Autodesk Inventor part; units mm, degrees
ref_plane "YZ Plane" through (0, 0, 0) normal (1, 0, 0) x (0, 1, 0)
ref_plane "XZ Plane" through (0, 0, 0) normal (0, 1, 0) x (-1, 0, 0)
ref_plane "XY Plane" through (0, 0, 0) normal (0, 0, 1) x (1, 0, 0)
sketch "Skizze1" plane through (0, 0, 0) normal (0, 0, 1) x (1, 0, 0)
  line L0 (-1.4434, 2.5) -> (1.4434, 2.5)
  line L1 (1.4434, 2.5) -> (2.8868, 0)
  line L2 (2.8868, 0) -> (1.4434, -2.5)
  line L3 (1.4434, -2.5) -> (-1.4434, -2.5)
  line L4 (-1.4434, -2.5) -> (-2.8868, 0)
  line L5 (-2.8868, 0) -> (-1.4434, 2.5)
  point P0 (0, 0)
  point P1 (0, 0)
  point P2 (0, 2.5)
  point P3 (0, -2.5)
  dimension "d3" = 120
  dimension "d4" = 120
  dimension "d5" = 120
  dimension "d6" = 5
extrude "Extrusion1" add sketch "Skizze1" along normal blind 5
sketch "Skizze2" plane through (0, 0, 5) normal (0, 0, 1) x (1, 0, 0)
  point P0 (0, 0)
  point P1 (0, 0)
hole "Bohrung1" at (0, 0, 5) direction (0, 0, -1) diameter 2.5 depth 4 tip angle 118
thread "Gewinde1"
sketch "Skizze3" plane through (0, 0, 0) normal (0, 0, -1) x (-1, 0, 0)
  circle A0 centre (0, 0) radius 1.25
  dimension "d18" = 2.5
extrude "Extrusion2" add sketch "Skizze3" along normal blind 4
thread "Gewinde2"
properties part number "5mm_Außengewinde"
CAD build for the part. Positions are in the model's coordinates, mm. A direction names the side the tool comes from. Coordinates: 2 decimals unless noted, no trailing zeros. Loops run counter-clockwise (first coordinate to the right, second up) from the corner with the lowest first, then second, coordinate; pieces in that order, holes last. Notation, with made-up numbers: (5, -31) - (29, -31) arc R22 ccw to (29, -18) - close; hole circle Ø9 at (-29.75, 78). An arc over 180 degrees is marked (long way). Return JSON: item names as keys, results as strings.
1. Band-saw the part on B-B (z = 0.75). Give the cut face in (x, y), and give its area (3 significant figures).
Result:
{"outline": "(-2.89, 0) - (-1.44, -2.5) - (1.44, -2.5) - (2.89, 0) - (1.44, 2.5) - (-1.44, 2.5) - close; hole circle Ø1.67 at (0, 0)", "area": "19.5 mm2"}
2. Mould opens along Y. For faces 1 (the flat face through (1, 1, 5)), 2 (the cylindrical face through (1.22, 0.27, 2.97)), 3 (the conical face through (-0.19, -0.1, 0.38)), 4 (the flat face through (-2.175, 1.233, 2.465)) say: released by +Y, released by -Y, zero draft, split by the parting line, or undercut.
Result:
{"face 1": "zero draft", "face 2": "undercut", "face 3": "undercut", "face 4": "released by +Y"}
3. Drop flat-ended pins along their axis: pin 1 (2 mm diameter, centred on y = -1.5, z = -2.5, fed in from +X); pin 2 (1.5 mm diameter, centred on x = -0.5, y = 0.5, fed in from +Z); pin 3 (1.5 mm diameter, centred on y = 1.5, z = 1, fed in from -X). Give the stop position or say it passes through.
Result:
{"pin 1": "stops at x = 1.15", "pin 2": "stops at z = 5", "pin 3": "stops at x = -2.45"}
4. Band-saw the part on A-A (z = 3). Give the cut face in (x, y), and give its area (3 significant figures).
Result:
{"outline": "(-2.89, 0) - (-1.44, -2.5) - (1.44, -2.5) - (2.89, 0) - (1.44, 2.5) - (-1.44, 2.5) - close; hole circle Ø2.5 at (0, 0)", "area": "16.7 mm2"}
5. Band-saw the part on C-C (y = 2.1). Give the cut face in (x, z).
Result:
{"outline": "(-1.67, 0) - (1.67, 0) - (1.67, 5) - (-1.67, 5) - close"}
6. 3-axis set-ups, long thin cutter, end or side, ignore diameter. For faces 5 (the flat face through (2.175, -1.233, 2.465)), 6 (the flat face through (1, 1, 0)): which of +Z, -Z, +X, -X, +Y, -Y reach the whole face in a straight line?
Result:
{"face 5": "+Z, -Z, +X, -Y", "face 6": "-Z"}
7. Probe L1, parallel to Y at x = 0, z = 2.25; L2, parallel to X at y = -0.3, z = 3.25; L3, parallel to Z at x = -2, y = -0.85. List the from-to ranges inside material, lowest first. Write a range as from..to.
Result:
{"L1": "y = -2.5..-1.25, 1.25..2.5", "L2": "x = -2.71..-1.21, 1.21..2.71", "L3": "z = 0..5"}
8. Band-saw the part on D-D (z = -1.25). Give the cut face in (x, y), and give its area (3 significant figures).
Result:
{"outline": "circle Ø2.5 at (0, 0)", "area": "4.91 mm2"}
